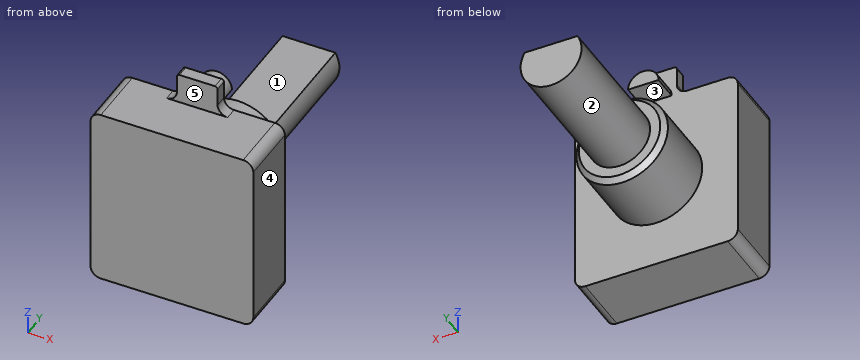
from build123d import *

# Parameters (mm, degrees)
SKETCH_1_W      = 16
SKETCH_1_H      = 18
EXTRUDE_1_DEPTH = 6
FILLET_1_R      = 1
SKETCH_2_W      = 4
SKETCH_2_H      = 1.2
EXTRUDE_2_DEPTH = 3
FILLET_2_R      = 1
FILLET_3_R      = 0.25
SKETCH_3_R      = 4.5
EXTRUDE_3_DEPTH = 7
CHAMFER_1_SIZE  = 0.5
EXTRUDE_4_DEPTH = 13
EXTRUDE_5_DEPTH = 2.5


with BuildPart() as part:
    # Эскиз1 → Бобышка-Вытянуть1 (new body)
    with BuildSketch(Plane(origin=(0, 0, 0), x_dir=(1, 0, 0), z_dir=(0, 1, 0))):
        Rectangle(SKETCH_1_W, SKETCH_1_H)
    extrude(amount=EXTRUDE_1_DEPTH)

    # Скругление1
    fillet_1_edges = [part.edges().sort_by_distance(p)[0] for p in [
        (8, 3, 9),
        (-8, 3, 9),
        (-8, 3, -9),
        (8, 3, -9),
    ]]
    fillet(fillet_1_edges, radius=FILLET_1_R)

    # Эскиз2 → Бобышка-Вытянуть2 (add)
    with BuildSketch(Plane.XY.offset(9)):
        with Locations((0, 5.4)):
            Rectangle(SKETCH_2_W, SKETCH_2_H)
    extrude(amount=EXTRUDE_2_DEPTH)

    # Скругление2
    fillet_2_edges = [part.edges().sort_by_distance(p)[0] for p in [
        (2, 5.4, 9),
        (-2, 5.4, 9),
    ]]
    fillet(fillet_2_edges, radius=FILLET_2_R)

    # Скругление3
    fillet_3_edges = [part.edges().sort_by_distance(p)[0] for p in [
        (2, 5.4, 12),
        (-2, 5.4, 12),
    ]]
    fillet(fillet_3_edges, radius=FILLET_3_R)

    # Эскиз3 → Бобышка-Вытянуть3 (add)
    with BuildSketch(Plane(origin=(0, 6, 0), x_dir=(1, 0, 0), z_dir=(0, 1, 0))):
        with Locations(Location((0, 0, 0), (0, 0, 270))):
            Circle(SKETCH_3_R)
    extrude(amount=EXTRUDE_3_DEPTH)

    # Фаска1
    chamfer_1_edges = [part.edges().sort_by_distance(p)[0] for p in [
        (0, 13, -4.5),
    ]]
    chamfer(chamfer_1_edges, length=CHAMFER_1_SIZE)

    # Эскиз4 → Бобышка-Вытянуть4 (add)
    with BuildSketch(Plane(origin=(0, 13, 0), x_dir=(1, 0, 0), z_dir=(0, 1, 0))):
        with BuildLine():
            Line((-2.598076211, -1.5), (2.598076211, -1.5))
            ThreePointArc((2.598076211, -1.5), (0, 3), (-2.598076211, -1.5))
        make_face()
    extrude(amount=EXTRUDE_4_DEPTH)

    # Эскиз5 → Бобышка-Вытянуть5 (add)
    with BuildSketch(Plane(origin=(0, 6, 0), x_dir=(1, 0, 0), z_dir=(0, 1, 0))):
        with BuildLine():
            Line((-1.5, -9), (1.5, -9))
            ThreePointArc((1.5, -9), (0, -10.5), (-1.5, -9))
        make_face()
    extrude(amount=EXTRUDE_5_DEPTH)


solid = part.part
Work out the finished part from the listing and answer in its coordinate system (mm). Face numbers are marked on the shaded views. A direction names the side the tool comes from. Round coordinates to 2 decimals unless told otherwise and drop trailing zeros. Order: outer loops, then holes, each group sorted by start corner. A loop starts at its lowest first (then second) coordinate and runs counter-clockwise, first axis right, second up. Notation, with made-up numbers: M 31,26 L 40,26 A25 ccw 40,58 Z; hole C 85.5,-6 d3. An arc over 180 degrees is marked long. One line per item, written item: value.
Q1. Find section C-C on y = 3.75. Write down the section's boundary in (x, z).
Derived:
outline: M -8,-8 A1 ccw -7,-9 L 7,-9 A1 ccw 8,-8 L 8,8 A1 ccw 7,9 L -7,9 A1 ccw -8,8 Z
Q2. Find section A-A on z = 0. Write down the section's boundary in (x, y), then the cut area to 3 significant figures.
Derived:
outline: M -8,0 L 8,0 L 8,6 L 4.5,6 L 4.5,12.5 L 4,13 L 3,13 L 3,26 L -3,26 L -3,13 L -4,13 L -4.5,12.5 L -4.5,6 L -8,6 Z
area: 237 mm²
Q3. Flat-ended cylindrical pins translate along their axes: pin 1 (12 mm diameter, centred on y = 15, z = 1, fed in from -X); pin 2 (1 mm diameter, centred on y = 7.5, z = 6, fed in from -X) (3 decimals); pin 3 (0.6 mm diameter, centred on y = 5.5, z = 11, fed in from +X); pin 4 (0.6 mm diameter, centred on y = 5.5, z = 11.5, fed in from -X). Find the tip coordinate at first contact, or state that the pin passes through.
Derived:
pin 1: x = -4.5
pin 2: through
pin 3: x = 2
pin 4: x = -2
Q4. For the marked faces 1, 2, 3, 4 and 5, determine the directions among +Z, -Z, +X, -X, +Y, -Y from which every point of the face is accessible in a straight line to the end or side of a thin tool.
Derived:
face 1: +Z, +X, -X, +Y
face 2: +Y
face 3: +X, -X, +Y
face 4: +Z, -Z, +X, +Y, -Y
face 5: +Z, +X, -X, -Y
Q5. Straight lines are drawn through the part: line 1 (Z direction, x = -0.75, y = 3.25); line 2 (Y direction, x = -5.25, z = 1.75); line 3 (Z direction, x = 2.5, y = 8.25). For each, find the intervals that lie inside material, in ascending order.
Derived:
line 1: -9 to 9
line 2: 0 to 6
line 3: -3.74 to 3.74
Q6. Find section B-B on x = 0. Write down the section's boundary in (y, z).
Derived:
outline: M 0,-9 L 6,-9 L 6,-4.5 L 12.5,-4.5 L 13,-4 L 13,-3 L 26,-3 L 26,1.5 L 13,1.5 L 13,4 L 12.5,4.5 L 6,4.5 L 6,9 L 8.5,9 L 8.5,10.5 L 6,10.5 L 6,12 L 4.8,12 L 4.8,9 L 0,9 Z
Q7. Find section D-D on x = 6.25. Write down the section's boundary in (y, z).
Derived:
outline: M 0,-9 L 6,-9 L 6,9 L 0,9 Z
